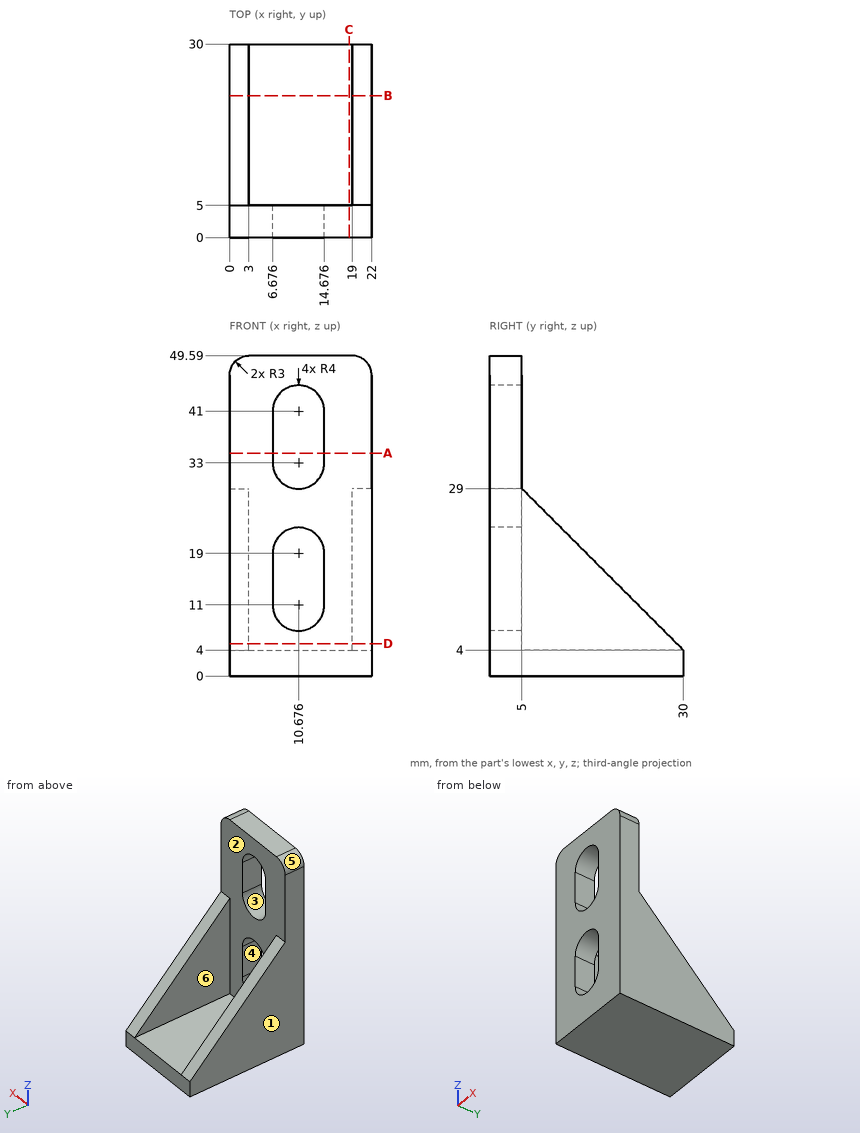
Could you check a few things on this drawing? It's one solid part, dimensions in mm from its lowest x, y, z. A direction names the side the tool comes from. Coordinates: 2 decimals unless noted, no trailing zeros. Order: outer loops, then holes, each group sorted by start corner. A loop starts at its lowest first (then second) coordinate and runs counter-clockwise, first axis right, second up.
1. If we section it at B-B (y = 22): Please give me the cut outline in (x, z), then the cut area to 3 significant figures.
2. I need wall thicknesses on line 1 (X direction, y = 13.5, z = 18); line 2 (Y direction, x = 4, z = 20.5); line 3 (Z direction, x = 4, y = 28.5). Which ranges of each line are inside material? Lowest first, please.
3. For the marked faces 1, 2 and 3, which set-ups out of +Z, -Z, +X, -X, +Y, -Y let a thin tool reach every point of the face, with its end or its side?
4. If we section it at A-A (z = 34.5): Please give me the cut outline in (x, y) (1 decimal), then the cut area to 3 significant figures.
5. Thinking about a two-plate mould opening in Z: for the marked faces 4, 5 and 6, which applies, +Z half, -Z half, draft (parallel to the pull), parting line (faces both ways), or undercut?
6. If we section it at C-C (x = 18.5): Please give me the cut outline in (y, z).
7. I'm going to push flat-ended pins straight in: pin 1 (11 mm diameter, centred on x = 9.5, z = 17, fed in from +Y); pin 2 (4 mm diameter, centred on x = 16.5, y = 26.5, fed in from +Z). Where does each tip first touch, or does it pass through?
8. If we section it at D-D (z = 5): Please give me the cut outline in (x, y).
Entries:
1. outline: (0, 0) - (22, 0) - (22, 12) - (19, 12) - (19, 4) - (3, 4) - (3, 12) - (0, 12) - close
1. area: 136 mm2
2. line 1: x = 0 to 3, 19 to 22
2. line 2: y = 0 to 5
2. line 3: z = 0 to 4
3. face 1: +Z, -Z, -X, +Y, -Y
3. face 2: +Z, +Y
3. face 3: +Y, -Y
4. outline: (0, 0) - (6.7, 0) - (6.7, 5) - (0, 5) - close; (14.7, 0) - (22, 0) - (22, 5) - (14.7, 5) - close
4. area: 70.0 mm2
5. face 4: undercut
5. face 5: +Z half
5. face 6: draft
6. outline: (0, 0) - (30, 0) - (30, 4) - (5, 4) - (5, 49.59) - (0, 49.59) - close
7. pin 1: stops at y = 5
7. pin 2: stops at z = 4
8. outline: (0, 0) - (22, 0) - (22, 29) - (19, 29) - (19, 5) - (3, 5) - (3, 29) - (0, 29) - close
